For this review, take the finished solid that the model builds, in its own axes (mm). A direction names the side the tool comes from. Round coordinates to 2 decimals unless told otherwise and drop trailing zeros. Order: outer loops, then holes, each group sorted by start corner. A loop starts at its lowest first (then second) coordinate and runs counter-clockwise, first axis right, second up. Notation, with made-up numbers: M 70.5,67 L 129.5,67 A14 cw 129.5,82 Z; hole C -33.75,-13 d11. An arc over 180 degrees is marked long. Answer as a JSON object with one key per item and string values.
from build123d import *

# Parameters (mm, degrees)
SKETCH2_R                            = 11
SKETCH2_R_2                          = 10
BOSS_EXTRUDE1_REACH                  = 445.723
BOSS_EXTRUDE1_END_RADIUS             = 11
SKETCH3_R                            = 11
SKETCH3_R_2                          = 10
BOSS_EXTRUDE1_DIRECTION_2_REACH      = 445.723
BOSS_EXTRUDE1_DIRECTION_2_END_RADIUS = 11
SKETCH5_R                            = 2.5
CUT_EXTRUDE1_DEPTH                   = 200
SKETCH6_R                            = 2.5
CUT_EXTRUDE2_DEPTH                   = 200


with BuildPart() as part:
    # Sweep1: sweep along a path in Sketch1
    with BuildLine(Plane.XY) as sweep1_path:
        Line((204, -388), (204, -82.797389364))
        ThreePointArc((204, -82.797389364), (196.899346401, -56.297389364), (177.5, -36.898042963))
        Line((177.5, -36.898042963), (125.889407689, -7.100653599))
        ThreePointArc((125.889407689, -7.100653599), (113.10681708, -1.805931207), (99.389407689, 0))
        Line((99.389407689, 0), (-99.389407689, 0))
        ThreePointArc((-99.389407689, 0), (-113.10681708, -1.805931207), (-125.889407689, -7.100653599))
        Line((-125.889407689, -7.100653599), (-177.5, -36.898042963))
        ThreePointArc((-177.5, -36.898042963), (-196.899346401, -56.297389364), (-204, -82.797389364))
        Line((-204, -82.797389364), (-204, -388))
    # Sketch2 → Sweep1 (sweep)
    with BuildSketch(Plane(origin=(204, -388, 0), x_dir=(-1, 0, 0), z_dir=(0, -1, 0))):
        Circle(SKETCH2_R)
        Circle(SKETCH2_R_2, mode=Mode.SUBTRACT)
    sweep(path=sweep1_path.line)

    # Boss-Extrude1: up to this cylinder (the profile starts outside it)
    boss_extrude1_end = Plane(origin=(204, -359.399207, 0), z_dir=(0, -1, 0)) * Cylinder(BOSS_EXTRUDE1_END_RADIUS, 914.446, mode=Mode.PRIVATE)
    # Sketch3 → Boss-Extrude1 (add, up to the surface)
    with BuildSketch(Plane(origin=(0, 0, 0), x_dir=(0, 0, -1), z_dir=(1, 0, 0)), mode=Mode.PRIVATE) as boss_extrude1_sk1:
        with Locations(Location((0, -359.399206555, 0), (0, 0, 180))):
            Circle(SKETCH3_R)
        with Locations(Location((0, -359.399206555, 0), (0, 0, 180))):
            Circle(SKETCH3_R_2, mode=Mode.SUBTRACT)
    boss_extrude1_tool1 = extrude(boss_extrude1_sk1.sketch, amount=BOSS_EXTRUDE1_REACH, mode=Mode.PRIVATE) - boss_extrude1_end
    add(boss_extrude1_tool1.solids().sort_by_distance((0, -359.399207, -10.688873))[0])

    # Boss-Extrude1 direction 2: up to this cylinder (the profile starts outside it)
    boss_extrude1_direction_2_end = Plane(origin=(-204, -359.399207, 0), z_dir=(0, 1, 0)) * Cylinder(BOSS_EXTRUDE1_DIRECTION_2_END_RADIUS, 914.446, mode=Mode.PRIVATE)
    # Sketch3 → Boss-Extrude1 direction 2 (add, up to the surface)
    with BuildSketch(Plane(origin=(0, 0, 0), x_dir=(0, 0, -1), z_dir=(1, 0, 0)), mode=Mode.PRIVATE) as boss_extrude1_direction_2_sk1:
        with Locations(Location((0, -359.399206555, 0), (0, 0, 180))):
            Circle(SKETCH3_R)
        with Locations(Location((0, -359.399206555, 0), (0, 0, 180))):
            Circle(SKETCH3_R_2, mode=Mode.SUBTRACT)
    boss_extrude1_direction_2_tool1 = extrude(boss_extrude1_direction_2_sk1.sketch, amount=-BOSS_EXTRUDE1_DIRECTION_2_REACH, mode=Mode.PRIVATE) - boss_extrude1_direction_2_end
    add(boss_extrude1_direction_2_tool1.solids().sort_by_distance((0, -359.399207, -10.688873))[0])

    # Sketch5 → Cut-Extrude1 (cut)
    with BuildSketch(Plane(origin=(-204, -388, 0), x_dir=(0, 0, 1), z_dir=(-1, 0, 0))):
        with Locations(Location((0, 57, 0), (0, 0, 90))):
            Circle(SKETCH5_R)
    cut_extrude1 = extrude(amount=CUT_EXTRUDE1_DEPTH, mode=Mode.SUBTRACT)

    # Sketch6 → Cut-Extrude2 (cut, symmetric)
    with BuildSketch(Plane(origin=(-204, -388, 0), x_dir=(0, 0, 1), z_dir=(-1, 0, 0))):
        with Locations(Location((0, 277, 0), (0, 0, 180))):
            Circle(SKETCH6_R)
    cut_extrude2 = extrude(amount=CUT_EXTRUDE2_DEPTH, both=True, mode=Mode.SUBTRACT)

    # Mirror1: Cut-Extrude1, Cut-Extrude2 across plane
    add(cut_extrude1.mirror(Plane(origin=(0, 0, 0), x_dir=(0, 0, 1), z_dir=(1, 0, 0))), mode=Mode.SUBTRACT)
    add(cut_extrude2.mirror(Plane(origin=(0, 0, 0), x_dir=(0, 0, 1), z_dir=(1, 0, 0))), mode=Mode.SUBTRACT)


solid = part.part
1) Machinability: for faces 4 (the flat face through (-214, -388, 2)), 5 (the cylindrical face through (194.763, -233.262, -3.83)), 6 (the cylindrical face through (-215, -238, 0)), which of the approach directions +Z, -Z, +X, -X, +Y, -Y give a long, thin tool a straight path to every point of the face, cutting with its end or side? Answer none if there is none.
Geometry check:
{"face 4": "+Z, -Z, +X, -X, -Y", "face 5": "-Y", "face 6": "none"}
2) Add section A-A on y = -156.5. State the section outline as (x, z) points, and give its area (3 significant figures).
Geometry check:
{"outline": "C -204,0 d22; C 204,0 d22; hole C -204,0 d20; hole C 204,0 d20", "area": "132 mm²"}
3) Insertion check: P1, Ø4.5, axis at y = -331, z = 0, coming from the +X side; P2, Ø2, axis at x = 3, z = 8, coming from the -Y side; P3, Ø2, axis at y = -105, z = -5, coming from the -X side. Each pin has a flat end and moves straight along its axis. Give the tip position at first contact, or say it passes through.
Geometry check:
{"P1": "stops at x = 194.26", "P2": "stops at y = -367.88", "P3": "stops at x = -214.25"}
4) For L1, parallel to X at y = -292.5, z = 1.5; L2, parallel to X at y = -133, z = 0.25; L3, parallel to Y at x = 1.5, z = -7, list the stretches that pass through material, from the lowest coordinate up.
Geometry check:
{"L1": "x = -214.9 to -213.89, -194.11 to -193.1, 193.1 to 194.11, 213.89 to 214.9", "L2": "x = -215 to -214, -194 to -193, 193 to 194, 214 to 215", "L3": "y = -367.88 to -366.54, -352.26 to -350.91, -8.49 to -7.14, 7.14 to 8.49"}
5) Mouldability with a two-part tool opening along Y and no side actions: class faces 1 (the cylindrical face through (-157.55, -12.69, 0.48)), 2 (the cylindrical face through (-194.763, -237.535, -3.83)), 3 (the flat face through (194, -388, -2)) as +Y half, -Y half, draft (parallel to the pull), parting line (faces both ways), or undercut.
Geometry check:
{"face 1": "undercut", "face 2": "draft", "face 3": "-Y half"}
6) Add section B-B on x = -165. State how many separate pieces and enclosed holes the cut face has, and give its area (3 significant figures).
Geometry check:
{"separate pieces": "2", "enclosed holes": "2", "area": "142 mm²"}
